The listing builds one solid part. Answer for the finished solid, in the listing's coordinates (mm). A direction names the side the tool comes from. Coordinates: 2 decimals unless noted, no trailing zeros. Order: outer loops, then holes, each group sorted by start corner. A loop starts at its lowest first (then second) coordinate and runs counter-clockwise, first axis right, second up. Notation, with made-up numbers: (67.5, 39) -> (88.5, 39) arc R21 cw to (88.5, 53) -> close; hole circle Ø5 at (-23.75, 39.5). An arc over 180 degrees is marked (long way). Write each question's results on one line, items separated by ' | '. Start each with the question number.
(1) The part is cut by section B-B, the plane x = -33.75. Give the vertices of the cut face in (y, z).
(2) The part is cut by section A-A, the plane z = -4.5. Give the vertices of the cut face in (x, y), then the cut area to 3 significant figures.
(3) A tool of negligible diameter and unlimited length cuts with its end or side. For faces 1 (the face through (-23, 17, -0.5)), 2 (the face through (-36.554, 16.005, -4.164)), 3 (the face through (-10.067, 18, 2)), 4 (the face through (-23, 16.293, 2)), 5 (the face through (-23, 18.743, 2)), from which of +Z, -Z, +X, -X, +Y, -Y can it reach the whole face along a straight path? Write none if from no direction.
(4) Given pin 1 (0.5 mm diameter, centred on x = -22, z = 2, fed in from +Y); pin 2 (1 mm diameter, centred on x = -26.5, z = 0, fed in from -Y); pin 3 (3 mm diameter, centred on x = -21.5, y = 16, fed in from -Z), each flat-ended and moving along its own axis, determine where each tip first touches the part or whether it passes through.
(5) Straight lines are drawn through the part: L1, parallel to Y at x = -36.85, z = -4.5; L2, parallel to X at y = 20.25, z = -4; L3, parallel to Z at x = -12.75, y = 19.25. For each, find the intervals that lie inside material, in ascending order.
(6) The part is cut by section C-C, the plane z = -5.75. Give the vertices of the cut face in (x, y), then the cut area to 3 significant figures.
(7) Determine the mould class of faces 6 (the face through (-37.467, 18, -2)), 7 (the face through (-35.667, 17.5, -2.7)), 8 (the face through (-36.6, 17.6, -8.5)) for opening direction X: +X half, -X half, draft (parallel to the pull), parting line (faces both ways), or undercut.
```python
from build123d import *

# Parameters (mm, degrees)
CROQUIS1_W                 = 26.4
CROQUIS1_H                 = 2.95
SALIENTE_EXTRUIR1_DEPTH    = 1.5
SALIENTE_EXTRUIR2_DEPTH    = 1
SALIENTE_EXTRUIR3_START    = 1
SALIENTE_EXTRUIR3_DEPTH    = 1
CROQUIS5_W                 = 26.4
CROQUIS5_H                 = 0.387649526
SALIENTE_EXTRUIR4_DEPTH    = 2.95
CROQUIS7_R                 = 1.5
CORTAR_EXTRUIR1_DEPTH      = 51
CORTAR_EXTRUIR2_START      = 26.4
CROQUIS8_R                 = 3
CORTAR_EXTRUIR2_DEPTH      = 26.4
CROQUIS9_W                 = 0.5
CROQUIS9_H                 = 1
SALIENTE_EXTRUIR5_DEPTH    = 20
CROQUIS11_W                = 1
CROQUIS11_H                = 1.007194245
CROQUIS11_H_2              = 16.042805755
CORTAR_EXTRUIR3_DEPTH      = 40
CROQUIS13_W                = 25.4
CROQUIS13_H                = 2.45
SALIENTE_EXTRUIR6_DEPTH    = 1
CROQUIS14_W                = 4.527159606
CROQUIS14_H                = 1.589204257
CROQUIS14_W_2              = 3.32574087
CROQUIS14_H_2              = 2.189079922
CORTAR_EXTRUIR4_DEPTH      = 21
CORTAR_EXTRUIR5_DEPTH      = 21
CORTAR_EXTRUIR5_DEPTH_BACK = 21
CROQUIS16_W                = 34.398488571
CROQUIS16_H                = 9.421589472
CROQUIS17_W                = 29.4
CROQUIS17_H                = 6.45
SALIENTE_EXTRUIR7_DEPTH    = 2
CROQUIS18_R                = 1.55
SALIENTE_EXTRUIR8_DEPTH    = 29.4
CORTAR_EXTRUIR6_DEPTH      = 12
CORTAR_EXTRUIR6_DEPTH_BACK = 32
CROQUIS19_W                = 25.8
CROQUIS19_H                = 10.578979108


with BuildPart() as part:
    # Croquis1 → Saliente-Extruir1 (new body)
    with BuildSketch(Plane.XY):
        with Locations((-22.767073783, 17.517805755)):
            Rectangle(CROQUIS1_W, CROQUIS1_H)
    extrude(amount=SALIENTE_EXTRUIR1_DEPTH)

    # Croquis2 → Saliente-Extruir2 (add)
    with BuildSketch(Plane(origin=(-9.567073783, 0, 0), x_dir=(0, 0, -1), z_dir=(1, 0, 0))):
        with BuildLine():
            Line((0, 18.992805755), (0.387649526, 18.992805755))
            ThreePointArc((0.387649526, 18.992805755), (6, 17.517805755), (0.387649526, 16.042805755))
            Line((0.387649526, 16.042805755), (0, 16.042805755))
            Line((0, 16.042805755), (-0.5, 16.042805755))
            Line((-0.5, 16.042805755), (-0.5, 18.992805755))
            Line((-0.5, 18.992805755), (0, 18.992805755))
        make_face()
    extrude(amount=SALIENTE_EXTRUIR2_DEPTH)

    # Croquis3 → Saliente-Extruir3 (add)
    with BuildSketch(Plane.ZY.offset(35.967073783).offset(SALIENTE_EXTRUIR3_START)):
        with BuildLine():
            Line((0.5, 18.992805755), (-0.387649526, 18.992805755))
            ThreePointArc((-0.387649526, 18.992805755), (-6, 17.517805755), (-0.387649526, 16.042805755))
            Line((-0.387649526, 16.042805755), (0.5, 16.042805755))
            Line((0.5, 16.042805755), (0.5, 18.992805755))
        make_face()
    extrude(amount=-SALIENTE_EXTRUIR3_DEPTH)

    # Croquis5 → Saliente-Extruir4 (add)
    with BuildSketch(Plane(origin=(0, 18.992805755, 0), x_dir=(1, 0, 0), z_dir=(0, 1, 0))):
        with Locations((-22.767073783, 0.193824763)):
            Rectangle(CROQUIS5_W, CROQUIS5_H)
    extrude(amount=-SALIENTE_EXTRUIR4_DEPTH)

    # Croquis7 → Cortar-Extruir1 (cut)
    with BuildSketch(Plane(origin=(-8.567073783, 0, 0), x_dir=(0, 0, -1), z_dir=(1, 0, 0))):
        with Locations(Location((3, 17.517805755, 0), (0, 0, 180))):
            Circle(CROQUIS7_R)
    extrude(amount=-CORTAR_EXTRUIR1_DEPTH, mode=Mode.SUBTRACT)

    # Croquis8 → Cortar-Extruir2 (cut)
    with BuildSketch(Plane.ZY.offset(9.567073783).offset(CORTAR_EXTRUIR2_START)):
        with Locations((-3, 17.517805755)):
            Circle(CROQUIS8_R)
    extrude(amount=-CORTAR_EXTRUIR2_DEPTH, mode=Mode.SUBTRACT)

    # Croquis9 → Saliente-Extruir5 (add)
    with BuildSketch(Plane(origin=(0, 0, 0), x_dir=(1, 0, 0), z_dir=(0, 1, 0))):
        with Locations((-37.017073783, -1)):
            Rectangle(CROQUIS9_W, CROQUIS9_H)
        with Locations((-8.518741189, -1)):
            Rectangle(CROQUIS9_W, CROQUIS9_H)
    extrude(amount=SALIENTE_EXTRUIR5_DEPTH)

    # Croquis11 → Cortar-Extruir3 (cut)
    with BuildSketch(Plane.ZY.offset(37.267073783)):
        with Locations((1, 19.496402878)):
            Rectangle(CROQUIS11_W, CROQUIS11_H)
        with Locations((1, 8.021402877)):
            Rectangle(CROQUIS11_W, CROQUIS11_H_2)
    extrude(amount=-CORTAR_EXTRUIR3_DEPTH, mode=Mode.SUBTRACT)

    # Croquis13 → Saliente-Extruir6 (add)
    with BuildSketch(Plane.XY.offset(1.5)):
        with Locations((-22.767073783, 17.517805755)):
            Rectangle(CROQUIS13_W, CROQUIS13_H)
    extrude(amount=SALIENTE_EXTRUIR6_DEPTH)

    # Croquis14 → Cortar-Extruir4 (cut)
    with BuildSketch(Plane(origin=(0, 18.992805755, 0), x_dir=(1, 0, 0), z_dir=(0, 1, 0))):
        with Locations((-38.230653586, -1.294602129)):
            Rectangle(CROQUIS14_W, CROQUIS14_H)
        with Locations((-7.904203348, -1.594539961)):
            Rectangle(CROQUIS14_W_2, CROQUIS14_H_2)
    extrude(amount=-CORTAR_EXTRUIR4_DEPTH, mode=Mode.SUBTRACT)

    # Croquis16 → Cortar-Extruir5 (cut, two sides: drawn at the far end of the back side and taken through both)
    with BuildSketch(Plane(origin=(0, 18.992805755, 0), x_dir=(1, 0, 0), z_dir=(0, 1, 0)).offset(-CORTAR_EXTRUIR5_DEPTH_BACK)):
        with Locations((-24.715099431, 3.210794736)):
            Rectangle(CROQUIS16_W, CROQUIS16_H)
    extrude(amount=CORTAR_EXTRUIR5_DEPTH + CORTAR_EXTRUIR5_DEPTH_BACK, mode=Mode.SUBTRACT)

    # Croquis17 → Saliente-Extruir7 (add)
    with BuildSketch(Plane(origin=(0, 0, 1.5), x_dir=(-1, 0, 0), z_dir=(0, 0, -1))):
        with Locations((22.767073783, 17.517805755)):
            Rectangle(CROQUIS17_W, CROQUIS17_H)
    extrude(amount=SALIENTE_EXTRUIR7_DEPTH)

    # Croquis18 → Saliente-Extruir8 (add)
    with BuildSketch(Plane(origin=(-8.067073783, 0, 0), x_dir=(0, 0, -1), z_dir=(1, 0, 0))):
        with BuildLine():
            Line((0.5, 20.742805755), (3.55055626, 21.40349187))
            ThreePointArc((3.55055626, 21.40349187), (8.5, 17.517805755), (3.55055626, 13.63211964))
            Line((3.55055626, 13.63211964), (0.5, 14.292805755))
            Line((0.5, 14.292805755), (0.5, 20.742805755))
        make_face()
        with Locations((4.5, 17.517805755)):
            Circle(CROQUIS18_R, mode=Mode.SUBTRACT)
    extrude(amount=-SALIENTE_EXTRUIR8_DEPTH)

    # Croquis19 → Cortar-Extruir6 (cut, two sides: drawn at the far end of the back side and taken through both)
    with BuildSketch(Plane(origin=(0, 20.742805755, 0), x_dir=(1, 0, 0), z_dir=(0, 1, 0)).offset(-CORTAR_EXTRUIR6_DEPTH_BACK)):
        with Locations((-22.767073783, 5.789489554)):
            Rectangle(CROQUIS19_W, CROQUIS19_H)
    extrude(amount=CORTAR_EXTRUIR6_DEPTH + CORTAR_EXTRUIR6_DEPTH_BACK, mode=Mode.SUBTRACT)


solid = part.part
```
Established:
1) outline: (14.29, -0.5) -> (20.74, -0.5) -> (20.74, 1.5) -> (18.74, 1.5) -> (18.74, 2.5) -> (16.29, 2.5) -> (16.29, 1.5) -> (14.29, 1.5) -> close
2) outline: (-37.47, 13.52) -> (-35.67, 13.52) -> (-35.67, 15.97) -> (-37.47, 15.97) -> close; (-37.47, 19.07) -> (-35.67, 19.07) -> (-35.67, 21.52) -> (-37.47, 21.52) -> close; (-9.87, 13.52) -> (-8.07, 13.52) -> (-8.07, 15.97) -> (-9.87, 15.97) -> close; (-9.87, 19.07) -> (-8.07, 19.07) -> (-8.07, 21.52) -> (-9.87, 21.52) -> close | area: 17.6 mm^2
3) face 1: -Z, +Y, -Y | face 2: +X, -X | face 3: +Z, +X, +Y, -Y | face 4: +Z, +X, -X, -Y | face 5: +Z, +X, -X, +Y
4) pin 1: stops at y = 18.74 | pin 2: stops at y = 14.29 | pin 3: stops at z = -0.5
5) L1: y = 13.52 to 15.97, 19.07 to 21.52 | L2: x = -37.47 to -35.67, -9.87 to -8.07 | L3: z = -0.5 to 1.5
6) outline: (-37.47, 13.72) -> (-35.67, 13.72) -> (-35.67, 16.6) -> (-37.47, 16.6) -> close; (-37.47, 18.43) -> (-35.67, 18.43) -> (-35.67, 21.32) -> (-37.47, 21.32) -> close; (-9.87, 13.72) -> (-8.07, 13.72) -> (-8.07, 16.6) -> (-9.87, 16.6) -> close; (-9.87, 18.43) -> (-8.07, 18.43) -> (-8.07, 21.32) -> (-9.87, 21.32) -> close | area: 20.8 mm^2
7) face 6: -X half | face 7: undercut | face 8: draft
